Read the model definition and answer for the solid it produces. Units are mm, in the model's axes. A direction names the side the tool comes from. Coordinates: 2 decimals unless noted, no trailing zeros. Order: outer loops, then holes, each group sorted by start corner. A loop starts at its lowest first (then second) coordinate and runs counter-clockwise, first axis right, second up. Notation, with made-up numbers: M 78.5,-15.75 L 92.5,-15.75 A21 cw 92.5,-11.75 Z; hole C 7,-9 d2. An arc over 180 degrees is marked long. Write each question's results on one line, items separated by ' | '.
```python
from build123d import *

# Parameters (mm, degrees)
ESQUISSE2_W                  = 3
ESQUISSE2_H                  = 6.625
ENL_V_MAT_EXTRU_1_DEPTH      = 10
ESQUISSE3_W                  = 1
ESQUISSE3_H                  = 19
ENL_V_MAT_EXTRU_2_DEPTH      = 18.363755354
ESQUISSE4_W                  = 9.5
ESQUISSE4_H                  = 1
ENL_V_MAT_EXTRU_3_DEPTH      = 7
ESQUISSE5_R                  = 1.25
ENL_V_MAT_EXTRU_4_DEPTH      = 10
ENL_V_MAT_EXTRU_6_REACH      = 21.5
ENL_V_MAT_EXTRU_6_END_RADIUS = 9.5
ESQUISSE7_R                  = 2


with BuildPart() as part:
    # Esquisse1 → Base-Révolution (revolve)
    with BuildSketch(Plane.XY, mode=Mode.PRIVATE) as base_r_volution_sk:
        Polygon((0, 1.5), (0, 9.5), (11, 9.5), (11, 3), (4, 3), (4, 1.5), align=None)
    revolve(base_r_volution_sk.sketch.rotate(Axis((0, 0, 0), (1, 0, 0)), 90), axis=Axis((0, 0, 0), (1, 0, 0)))

    # Esquisse2 → Enlèv. mat.-Extru.1 (cut, symmetric)
    with BuildSketch(Plane.XY):
        with Locations((1.5, 6.1875)):
            Rectangle(ESQUISSE2_W, ESQUISSE2_H)
        with Locations((1.5, -6.1875)):
            Rectangle(ESQUISSE2_W, ESQUISSE2_H)
    extrude(amount=ENL_V_MAT_EXTRU_1_DEPTH, both=True, mode=Mode.SUBTRACT)

    # Esquisse3 → Enlèv. mat.-Extru.2 (cut, through all)
    with BuildSketch(Plane(origin=(0, 0, 0), x_dir=(1, 0, 0), z_dir=(0, 1, 0))):
        with Locations((4.5, 0)):
            Rectangle(ESQUISSE3_W, ESQUISSE3_H)
    extrude(amount=-ENL_V_MAT_EXTRU_2_DEPTH, mode=Mode.SUBTRACT)

    # Esquisse4 → Enlèv. mat.-Extru.3 (cut)
    with BuildSketch(Plane(origin=(11, 0, 0), x_dir=(0, 0, -1), z_dir=(1, 0, 0))):
        with Locations((-4.75, 0)):
            Rectangle(ESQUISSE4_W, ESQUISSE4_H)
    extrude(amount=-ENL_V_MAT_EXTRU_3_DEPTH, mode=Mode.SUBTRACT)

    # Esquisse5 → Enlèv. mat.-Extru.4 (cut, symmetric)
    with BuildSketch(Plane(origin=(0, 0, 0), x_dir=(1, 0, 0), z_dir=(0, 1, 0))):
        with Locations(Location((8, -6, 0), (0, 0, 270))):
            Circle(ESQUISSE5_R)
    extrude(amount=ENL_V_MAT_EXTRU_4_DEPTH, both=True, mode=Mode.SUBTRACT)

    # Enlèv. mat.-Extru.6: up to this cylinder (the profile starts inside it)
    enl_v_mat_extru_6_end = Plane(origin=(8, 0, 0), z_dir=(-1, 0, 0)) * Cylinder(ENL_V_MAT_EXTRU_6_END_RADIUS, 63, mode=Mode.PRIVATE)
    # Esquisse7 → Enlèv. mat.-Extru.6 (cut, up to the surface)
    with BuildSketch(Plane.XZ.offset(-3.5), mode=Mode.PRIVATE) as enl_v_mat_extru_6_sk1:
        with Locations(Location((8, 6, 0), (0, 0, 270))):
            Circle(ESQUISSE7_R)
    enl_v_mat_extru_6_tool1 = extrude(enl_v_mat_extru_6_sk1.sketch, amount=-ENL_V_MAT_EXTRU_6_REACH, mode=Mode.PRIVATE) & enl_v_mat_extru_6_end
    add(enl_v_mat_extru_6_tool1.solids().sort_by_distance((8, 3.5, 6))[0], mode=Mode.SUBTRACT)


solid = part.part
```
(1) The part is cut by section B-B, the plane y = -8.5. Write down the section's boundary in (x, z), then the cut area to 3 significant figures.
Conclusion:
outline: M 3,-4.24 L 4,-4.24 L 4,4.24 L 3,4.24 Z; M 5,-4.24 L 11,-4.24 L 11,4.24 L 5,4.24 Z | area: 59.4 mm²
(2) The part is cut by section A-A, the plane z = 0. Write down the section's boundary in (x, y) (3 decimals), then the cut area to 3 significant figures.
Conclusion:
outline: M 0,-2.875 L 3,-2.875 L 3,-9.5 L 4,-9.5 L 4,-1.5 L 0,-1.5 Z; M 0,1.5 L 4,1.5 L 4,3 L 11,3 L 11,9.5 L 3,9.5 L 3,2.875 L 0,2.875 Z; M 5,-9.5 L 11,-9.5 L 11,-3 L 5,-3 Z | area: 109 mm²
(3) For faces 1 (the flat face through (5, -5, 0)), 2 (the flat face through (1, 2.875, 0)), 3 (the flat face through (9.4, -0.5, 6.3)), determine the directions among +Z, -Z, +X, -X, +Y, -Y from which every point of the face is accessible in a straight line to the end or side of a thin tool.
Conclusion:
face 1: +Z, -Z, -Y | face 2: +Z, -Z, -X, +Y | face 3: +Z, +X
(4) The part is cut by section C-C, the plane z = 5.75. Write down the section's boundary in (x, y) (3 decimals), then the cut area to 3 significant figures.
Conclusion:
outline: M 0,-2.875 L 3,-2.875 L 3,-7.562 L 4,-7.562 L 4,0.5 L 6.775,0.5 L 6.775,3.5 L 6.016,3.5 L 6.016,7.562 L 3,7.562 L 3,2.875 L 0,2.875 Z; M 5,-7.562 L 6.775,-7.562 L 6.775,-0.5 L 5,-0.5 Z; M 9.225,-7.562 L 11,-7.562 L 11,-0.5 L 9.225,-0.5 Z; M 9.225,0.5 L 11,0.5 L 11,7.562 L 9.984,7.562 L 9.984,3.5 L 9.225,3.5 Z | area: 83.4 mm²
(5) Straight lines are drawn through the part: line 1 (X direction, y = -6.5, z = 6); line 2 (X direction, y = 5.6, z = 6); line 3 (Z direction, x = 8, y = -2.25). For each, find the intervals that lie inside material, in ascending order.
Conclusion:
line 1: 3 to 4, 5 to 6.75, 9.25 to 11 | line 2: 3 to 6, 10 to 11 | line 3: -9.23 to -1.98, 1.98 to 4.75, 7.25 to 9.23
(6) The mould has two halves that part along X. Classify faces 4 (the flat face through (3, 5, 0)), 5 (the flat face through (4.5, 0, -6.3)), 6 (the flat face through (1, -2.875, 0)): pulls with the +X half, pulls with the -X half, needs draft (parallel to the pull), parting line crosses it, or undercut.
Conclusion:
face 4: pulls with the -X half | face 5: undercut | face 6: needs draft
(7) The part is cut by section D-D, the plane x = 8. Write down the section's boundary in (y, z).
Conclusion:
outline: M -8.23,4.75 A9.5 ccw long 8.62,4 L 3.5,4 L 3.5,4.75 L 0.5,4.75 L 0.5,2.96 A3 cw long -0.5,2.96 L -0.5,4.75 Z; M -6.14,7.25 L -0.5,7.25 L -0.5,9.49 A9.5 ccw Z; M 0.5,7.25 L 3.5,7.25 L 3.5,8 L 5.12,8 A9.5 ccw 0.5,9.49 Z
(8) Given pin 1 (1 mm diameter, centred on x = 7, z = -1, fed in from -Y); pin 2 (6.5 mm diameter, centred on x = 7.5, z = 7, fed in from +Y); pin 3 (5.5 mm diameter, centred on y = -7, z = 3.5, fed in from -X), each flat-ended and moving along its own axis, determine where each tip first touches the part or whether it passes through.
Conclusion:
pin 1: y = -9.49 | pin 2: y = 8.73 | pin 3: x = 3
